Read the model definition and answer for the solid it produces. Units are mm, in the model's axes. Face numbers are marked on the shaded views. A direction names the side the tool comes from. Round coordinates to 2 decimals unless told otherwise and drop trailing zeros. Write each loop counter-clockwise with the first axis right and the second up, starting at its lowest first coordinate (ties: lowest second). Pieces come first, ordered by that corner, then holes. Notation, with made-up numbers: (44.25, 9) - (68.25, 9) arc R20 ccw to (68.25, 13) - close; hole circle Ø3 at (39.5, 76.5). An arc over 180 degrees is marked (long way). Use one line per item in the form item = value. Start each with the question number.
1) For the marked faces 1 and 2, determine the directions among +Z, -Z, +X, -X, +Y, -Y from which every point of the face is accessible in a straight line to the end or side of a thin tool.
2) For a pull along X with two mould halves and no side action, classify the marked faces 3, 4 and 5 as released by +X, released by -X, zero draft, split by the parting line, or undercut.
3) The part is cut by section A-A, the plane y = 13. Give the vertices of the cut face in (x, z), plus the area to 3 significant figures.
4) The part is cut by section C-C, the plane z = -41. Give the vertices of the cut face in (x, y), plus the area to 3 significant figures.
5) The part is cut by section D-D, the plane x = 62.5. Count the separate pieces of the cut face and the enclosed holes in it, plus the area to 3 significant figures.
6) Each of these flat-tipped pins is pushed along its axis until it touches: pin 1 (22.5 mm diameter, centred on x = 51.5, z = 62, fed in from +Y); pin 2 (8.5 mm diameter, centred on x = 53.5, z = -55.5, fed in from +Y). Where does it stop, or does it pass through?
7) The part is cut by section B-B, the plane x = -37. Give the vertices of the cut face in (y, z).
8) Consider line 1 along Z through (x, y) = (57, 22.5); line 2 along X through (y, z) = (17, -56.5); line 3 along Z through (x, y) = (62.5, 9). Determine where each line is inside the solid, lowest interval first. Write a range as from..to.
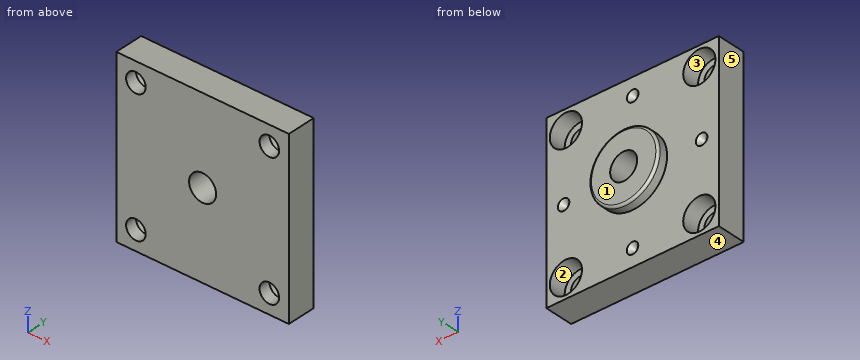
from build123d import *

# Parameters (mm, degrees)
IZIM2_W                     = 150
IZIM2_H                     = 150
Y_KSEKLIK_EKSTR_ZYON1_DEPTH = 25
IZIM3_R                     = 30
Y_KSEKLIK_EKSTR_ZYON2_DEPTH = 9
RADYUS1_R                   = 2
M25X1_5_DI_LI_DELIK2_D      = 23.5
DELIK1_D                    = 17
DELIK1_CBORE_D              = 28
DELIK1_CBORE_DEPTH          = 15
DAIRESEL_KAPLAMA2_COUNT     = 4


with BuildPart() as part:
    # Çizim2 → Yükseklik-Ekstrüzyon1 (new body)
    with BuildSketch(Plane(origin=(0, 0, 0), x_dir=(1, 0, 0), z_dir=(0, 1, 0))):
        Rectangle(IZIM2_W, IZIM2_H)
    extrude(amount=Y_KSEKLIK_EKSTR_ZYON1_DEPTH)

    # Çizim3 → Yükseklik-Ekstrüzyon2 (add)
    with BuildSketch(Plane(origin=(0, 25, 0), x_dir=(1, 0, 0), z_dir=(0, 1, 0))):
        with Locations(Location((0, 0, 0), (0, 0, 270))):
            Circle(IZIM3_R)
    extrude(amount=Y_KSEKLIK_EKSTR_ZYON2_DEPTH)

    # Radyus1
    radyus1_edges = [part.edges().sort_by_distance(p)[0] for p in [
        (0, 34, -30),
    ]]
    fillet(radyus1_edges, radius=RADYUS1_R)

    # M25x1.5 Dişli Delik2 (through all)
    with Locations(Plane(origin=(-0.00426246, 34, 0.065902754), x_dir=(0, 0, 1), z_dir=(0, 1, 0))):
        with Locations((0, 0)):
            Hole(M25X1_5_DI_LI_DELIK2_D / 2)

    # Delik1 (through all)
    with Locations(Plane(origin=(-57.998400022, 25, -57.998400022), x_dir=(0, 0, 1), z_dir=(0, 1, 0))):
        with Locations((0, 0), (0, 116), (116, 116), (116, 0)):
            CounterBoreHole(DELIK1_D / 2, DELIK1_CBORE_D / 2, DELIK1_CBORE_DEPTH)

    # Çizim8 → Kes-Döndür1 (revolve, cut)
    with BuildSketch(Plane.XY, mode=Mode.PRIVATE) as kes_d_nd_r1_sk:
        Polygon((-65, 25), (-60, 20), (-60, 25), align=None)
    kes_d_nd_r1 = revolve(kes_d_nd_r1_sk.sketch.rotate(Axis((-60, 20, 0), (0, 1, 0)), 90), axis=Axis((-60, 20, 0), (0, 1, 0)), mode=Mode.SUBTRACT)

    # Dairesel Kaplama2: Kes-Döndür1 ×4 about axis
    dairesel_kaplama2_axis = Axis((-0.00426246, 0, 0.065902754), (0, 1, 0))
    for i in range(1, DAIRESEL_KAPLAMA2_COUNT):
        add(kes_d_nd_r1.rotate(dairesel_kaplama2_axis, i * 360 / DAIRESEL_KAPLAMA2_COUNT), mode=Mode.SUBTRACT)


solid = part.part
Geometry results:
q1.face_1 = +Z, -Z, +X, -X, +Y
q1.face_2 = +Y
q2.face_3 = undercut
q2.face_4 = zero draft
q2.face_5 = released by -X
q3.outline = (-75, -75) - (75, -75) - (75, 75) - (-75, 75) - close; hole circle Ø28 at (-58, -58); hole circle Ø28 at (-58, 58); hole circle Ø23.5 at (0, 0.07); hole circle Ø28 at (58, -58); hole circle Ø28 at (58, 58)
q3.area = 19,600 mm2
q4.outline = (-75, 0) - (75, 0) - (75, 25) - (-75, 25) - close
q4.area = 3,750 mm2
q5.separate_pieces = 3
q5.enclosed_holes = 0
q5.area = 2,650 mm2
q6.pin_1 = 25
q6.pin_2 = 10
q7.outline = (0, -75) - (25, -75) - (25, 75) - (0, 75) - close
q8.line_1 = -75..-71.96, -44.03..44.04, 71.97..75
q8.line_2 = -75..-71.92, -44.08..44.08, 71.92..75
q8.line_3 = -75..-65.21, -50.79..50.79, 65.21..75
